Check sheet for the modelled part. Datum: model origin and axes. Units: mm. Round coordinates to 2 decimals unless told otherwise and drop trailing zeros. Loops run counter-clockwise (first coordinate to the right, second up) from the corner with the lowest first, then second, coordinate; pieces in that order, holes last. Notation, with made-up numbers: (79.5, 36.25) -> (135.5, 36.25) arc R24 ccw to (135.5, 71.25) -> close; hole circle Ø10 at (24, -34.75). An arc over 180 degrees is marked (long way). Return JSON: item names as keys, results as strings.
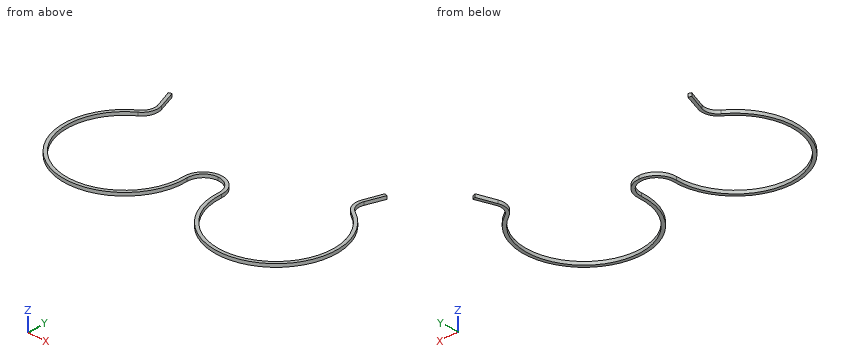
from build123d import *
from build123d.topology import SkipClean

# Parameters (mm, degrees)
BASE_EXTRUSION_DEPTH = 1


with BuildPart() as part:
    # Esquisse2 → Base-Extrusion (new body)
    with BuildSketch(Plane.XY):
        with BuildLine():
            Line((34.681264504, 26.422728636), (32.618025795, 20.754026872))
            ThreePointArc((32.618025795, 20.754026872), (32.588449466, 18.102034919), (34.224309969, 16.014477377))
            ThreePointArc((34.224309969, 16.014477377), (32.781477268, -16.8489067), (5.01650022, 0.791666667))
            ThreePointArc((5.01650022, 0.791666667), (3.629281566, 4.461093276), (0.020842383, 6))
            Line((0.020842383, 6), (0.020842383, 7))
            ThreePointArc((0.020842383, 7), (4.350969402, 5.153311931), (6.015631788, 0.75))
            ThreePointArc((6.015631788, 0.75), (32.285641023, -15.979616793), (33.750040286, 15.130654792))
            ThreePointArc((33.750040286, 15.130654792), (31.732063255, 17.702086165), (31.734019754, 20.970799485))
            Line((31.734019754, 20.970799485), (33.747574085, 26.781239692))
            ThreePointArc((33.747574085, 26.781239692), (34.215992075, 26.606080244), (34.681264504, 26.422728636))
        make_face()
    extrude(amount=-BASE_EXTRUSION_DEPTH)

    # Bossage-Symétrie1: part across plane


with BuildPart() as part_1:
    with SkipClean():  # the faces are left unmerged after this step: merging them gives an invalid solid
        add(part.part)
        add(part.part.mirror(Plane(origin=(0.020842383, 7, -1), x_dir=(0, 0, 1), z_dir=(-1, 0, 0))))


solid = part_1.part
Q1. Go/stop test with a flat-tipped pin: pin 1 (21.5 mm diameter, centred on x = 24, y = 0, fed in from +Z). Record where the tip stops, or that it passes through.
Results list:
{"pin 1": "through"}
Q2. Section check C-C (x = 24). Record the boundary of the cut face in (y, z).
Results list:
{"outline": "(-19, -1) -> (-18, -1) -> (-18, 0) -> (-19, 0) -> close"}
Q3. Section check D-D (x = 12.5). Record the boundary of the cut face in (y, z), then the cut area to 3 significant figures.
Results list:
{"outline": "(-15.12, -1) -> (-13.85, -1) -> (-13.85, 0) -> (-15.12, 0) -> close", "area": "1.28 mm^2"}
Q4. Section check B-B (z = -0.15). Record the boundary of the cut face in (x, y), then the cut area to 3 significant figures.
Results list:
{"outline": "(-34.64, 26.42) -> (-32.58, 20.75) arc R4 cw to (-34.18, 16.01) arc R19 ccw (long way) to (-4.97, 0.79) arc R5 cw (long way) to (5.02, 0.79) arc R19 ccw (long way) to (34.22, 16.01) arc R4 cw to (32.62, 20.75) -> (34.68, 26.42) arc R28.5 ccw to (33.75, 26.78) -> (31.73, 20.97) arc R5 ccw to (33.75, 15.13) arc R18 cw (long way) to (6.02, 0.75) arc R6 ccw (long way) to (-5.97, 0.75) arc R18 cw (long way) to (-33.71, 15.13) arc R5 ccw to (-31.69, 20.97) -> (-33.71, 26.78) arc R28.5 ccw to start", "area": "196 mm^2"}
Q5. Section check A-A (y = -5.5). Record the boundary of the cut face in (x, z).
Results list:
{"outline": "(-42.14, -1) -> (-41.1, -1) -> (-41.1, 0) -> (-42.14, 0) -> close; (-6.82, -1) -> (-5.77, -1) -> (-5.77, 0) -> (-6.82, 0) -> close; (5.81, -1) -> (6.86, -1) -> (6.86, 0) -> (5.81, 0) -> close; (41.14, -1) -> (42.19, -1) -> (42.19, 0) -> (41.14, 0) -> close"}
Q6. Material ranges on line 1 (X direction, y = 0, z = -0.3); line 2 (X direction, y = -3.5, z = -0.25); line 3 (X direction, y = 11.5, z = -0.75), recorded low to high.
Results list:
{"line 1": "-42.96 to -41.96, -5.96 to -4.96, 5 to 6, 42 to 43", "line 2": "-42.63 to -41.61, -6.3 to -5.28, 5.33 to 6.34, 41.66 to 42.67", "line 3": "-39.08 to -37.81, 37.85 to 39.12"}
